The listing builds one solid part. Answer for the finished solid, in the listing's coordinates (mm). A direction names the side the tool comes from. Give positions to 0.01 mm unless a question says otherwise; leave off trailing zeros. Write each loop counter-clockwise with the first axis right and the second up, starting at its lowest first coordinate (ties: lowest second). Pieces come first, ordered by that corner, then holes. Notation, with made-up numbers: (-39, 63) - (-35, 63) arc R12 ccw to (-35, 81) - close; hole circle Ø9 at (79.5, 70). An arc over 180 degrees is marked (long way). Return JSON: item names as keys, results as strings.
from build123d import *

# Parameters (mm, degrees)
SKICA1_W                 = 54.3
SKICA1_H                 = 104.3
SKICA1_W_2               = 51
SKICA1_H_2               = 101
P_IDAT_VYSUNUT_M1_DEPTH  = 1.2
SKICA2_W                 = 54.3
SKICA2_H                 = 104.3
P_IDAT_VYSUNUT_M2_DEPTH  = 20
SKICA3_R                 = 1.5
ODEBRAT_VYSUNUT_M1_DEPTH = 118.085631057
SKICA5_W                 = 8
SKICA5_H                 = 4
ODEBRAT_VYSUNUT_M2_DEPTH = 2
SKICA6_W                 = 10
SKICA6_H                 = 4
ODEBRAT_VYSUNUT_M3_DEPTH = 5
SKICA9_W                 = 15
SKICA9_H                 = 5
P_IDAT_VYSUNUT_M4_DEPTH  = 2
ZKOSEN_1_SIZE            = 2
SKICA10_W                = 15
SKICA10_H                = 5
P_IDAT_VYSUNUT_M5_DEPTH  = 3
ZKOSEN_2_SIZE            = 3
ZAOBLIT2_R               = 1
ZAOBLIT3_R               = 2
ODEBRAT_VYSUNUT_M5_DEPTH = 12.5
SKICA12_R                = 1.5
ODEBRAT_VYSUNUT_M6_DEPTH = 118.296568577


with BuildPart() as part:
    # Skica1 → Přidat vysunutím1 (new body)
    with BuildSketch(Plane(origin=(0, 0, 0), x_dir=(1, 0, 0), z_dir=(0, 1, 0))):
        with Locations((25.5, 50.5)):
            Rectangle(SKICA1_W, SKICA1_H)
        with Locations((25.5, 50.5)):
            Rectangle(SKICA1_W_2, SKICA1_H_2, mode=Mode.SUBTRACT)
    extrude(amount=P_IDAT_VYSUNUT_M1_DEPTH)

    # Skica2 → Přidat vysunutím2 (add)
    # profile 1 of 5: a face of its own
    with BuildSketch(Plane.XZ):
        with Locations((25.5, -50.5)):
            Rectangle(SKICA2_W, SKICA2_H)
        Polygon((0, -8), (0, 0), (8, 0), (43, 0), (51, 0), (51, -8), (51, -93), (51, -101), (43, -101), (8, -101), (0, -101), (0, -93), align=None, mode=Mode.SUBTRACT)
    # profile 2 of 5: a face of its own
    with BuildSketch(Plane.XZ):
        with BuildLine():
            Line((8, 0), (0, 0))
            Line((0, 0), (0, -8))
            ThreePointArc((0, -8), (5.656854249, -5.656854249), (8, 0))
        make_face()
    # profile 3 of 5: a face of its own
    with BuildSketch(Plane.XZ):
        with BuildLine():
            ThreePointArc((8, -101), (5.656854249, -95.343145751), (0, -93))
            Line((0, -93), (0, -101))
            Line((0, -101), (8, -101))
        make_face()
    # profile 4 of 5: a face of its own
    with BuildSketch(Plane.XZ):
        with BuildLine():
            Line((51, -101), (51, -93))
            ThreePointArc((51, -93), (45.343145751, -95.343145751), (43, -101))
            Line((43, -101), (51, -101))
        make_face()
    # profile 5 of 5: a face of its own
    with BuildSketch(Plane.XZ):
        with BuildLine():
            Line((51, 0), (43, 0))
            ThreePointArc((43, 0), (45.343145751, -5.656854249), (51, -8))
            Line((51, -8), (51, 0))
        make_face()
    extrude(amount=P_IDAT_VYSUNUT_M2_DEPTH)

    # Skica3 → Odebrat vysunutím1 (cut, through all)
    with BuildSketch(Plane(origin=(0, 0, 0), x_dir=(1, 0, 0), z_dir=(0, 1, 0))):
        with Locations(Location((3.5, 97.5, 0), (0, 0, 270))):
            Circle(SKICA3_R)
        with Locations(Location((47.5, 97.5, 0), (0, 0, 270))):
            Circle(SKICA3_R)
        with Locations(Location((47.5, 3.5, 0), (0, 0, 270))):
            Circle(SKICA3_R)
    extrude(amount=-ODEBRAT_VYSUNUT_M1_DEPTH, mode=Mode.SUBTRACT)

    # Skica5 → Odebrat vysunutím2 (cut)
    with BuildSketch(Plane(origin=(0, 0, 0), x_dir=(0, 0, -1), z_dir=(1, 0, 0))):
        with Locations((27, -8.6)):
            Rectangle(SKICA5_W, SKICA5_H)
    extrude(amount=-ODEBRAT_VYSUNUT_M2_DEPTH, mode=Mode.SUBTRACT)

    # Skica6 → Odebrat vysunutím3 (cut, symmetric)
    with BuildSketch(Plane(origin=(0, 0, 0), x_dir=(-1, 0, 0), z_dir=(0, 0, -1))):
        with Locations((-12, -9.2)):
            Rectangle(SKICA6_W, SKICA6_H)
    extrude(amount=ODEBRAT_VYSUNUT_M3_DEPTH, both=True, mode=Mode.SUBTRACT)

    # Skica9 → Přidat vysunutím4 (add)
    with BuildSketch(Plane.ZY.offset(-51)):
        with Locations((-56.5, -2.5)):
            Rectangle(SKICA9_W, SKICA9_H)
    extrude(amount=P_IDAT_VYSUNUT_M4_DEPTH)

    # Zkosení1
    zkosen_1_edges = [part.edges().sort_by_distance(p)[0] for p in [
        (49, -5, -56.5),
    ]]
    chamfer(zkosen_1_edges, length=ZKOSEN_1_SIZE - 0.0001)  # a hair under: the kernel refuses the full size

    # Skica10 → Přidat vysunutím5 (add)
    with BuildSketch(Plane(origin=(0, 0, 0), x_dir=(0, 0, -1), z_dir=(1, 0, 0))):
        with Locations((70.5, -2.5)):
            Rectangle(SKICA10_W, SKICA10_H)
    extrude(amount=P_IDAT_VYSUNUT_M5_DEPTH)

    # Zkosení2
    zkosen_2_edges = [part.edges().sort_by_distance(p)[0] for p in [
        (3, -5, -70.5),
    ]]
    chamfer(zkosen_2_edges, length=ZKOSEN_2_SIZE - 0.0001)  # a hair under: the kernel refuses the full size

    # Zaoblit2
    zaoblit2_edges = [part.edges().sort_by_distance(p)[0] for p in [
        (7, -11.2, -1.111491673),
        (17, -11.2, 0.825),
    ]]
    fillet(zaoblit2_edges, radius=ZAOBLIT2_R)

    # Zaoblit3
    zaoblit3_edges = [part.edges().sort_by_distance(p)[0] for p in [
        (-1.65, -9.4, -102.65),
        (52.65, -9.4, -102.65),
        (52.65, -9.4, 1.65),
        (-1.65, -9.4, 1.65),
    ]]
    fillet(zaoblit3_edges, radius=ZAOBLIT3_R)

    # Skica11 → Odebrat vysunutím5 (cut)
    with BuildSketch(Plane(origin=(0, 0, 0), x_dir=(1, 0, 0), z_dir=(0, 1, 0))):
        with BuildLine():
            Line((0, 8), (0, 0))
            Line((0, 0), (8, 0))
            ThreePointArc((8, 0), (5.656854249, 5.656854249), (0, 8))
        make_face()
    extrude(amount=-ODEBRAT_VYSUNUT_M5_DEPTH, mode=Mode.SUBTRACT)

    # Skica12 → Odebrat vysunutím6 (cut, through all)
    with BuildSketch(Plane.XZ.offset(20)):
        with Locations(Location((3.5, -3.5, 0), (0, 0, 270))):
            Circle(SKICA12_R)
    extrude(amount=-ODEBRAT_VYSUNUT_M6_DEPTH, mode=Mode.SUBTRACT)


solid = part.part
Item 1: For faces 4 (the face through (49, 0, -99)), 5 (the face through (1, -2, -78)), 6 (the face through (-1, 1.2, -51)), determine the directions among +Z, -Z, +X, -X, +Y, -Y from which every point of the face is accessible in a straight line to the end or side of a thin tool.
Answer below:
{"face 4": "+Y", "face 5": "+Y, -Y", "face 6": "+Z, -Z, +X, -X, +Y"}
Item 2: A cutting plane is placed at C-C on x = 9.5. Determine the outline of the cut face in (y, z).
Answer below:
{"outline": "(-20, -102.65) - (1.2, -102.65) - (1.2, -101) - (-20, -101) - close; (-20, 0) - (-11.2, 0) - (-11.2, 1.65) - (-20, 1.65) - close; (-7.2, 0) - (1.2, 0) - (1.2, 1.65) - (-7.2, 1.65) - close"}
Item 3: Flat-ended cylindrical pins translate along their axes: P1, Ø1.8, axis at y = -9, z = 1, coming from the +X side; P2, Ø5, axis at x = 47.5, z = -97.5, coming from the -Y side; P3, Ø6.5, axis at x = 45, z = -4, coming from the +Y side; P4, Ø0.5, axis at x = -1, y = -8, coming from the -Z side. Find the tip coordinate at first contact, or state that the pin passes through.
Answer below:
{"P1": "stops at x = 52.6", "P2": "stops at y = -20", "P3": "stops at y = 0", "P4": "stops at z = -102.32"}
Item 4: The mould has two halves that part along X. Classify faces 1 (the face through (-1.08, -9.55, -102.05)), 2 (the face through (2.17, -9.86, -96.81)), 3 (the face through (52.05, -9.25, 1.08)): +X half, -X half, draft (parallel to the pull), parting line (faces both ways), or undercut.
Answer below:
{"face 1": "-X half", "face 2": "undercut", "face 3": "+X half"}
Item 5: Consider L1, parallel to X at y = -10, z = -68.5; L2, parallel to Z at x = 26, y = -12.75; L3, parallel to X at y = -15.25, z = -97.5. Determine where each line is inside the solid, lowest interval first.
Answer below:
{"L1": "x = -1.65 to 0, 51 to 52.65", "L2": "z = -102.65 to -101, 0 to 1.65", "L3": "x = -1.65 to 2, 5 to 7.19, 43.81 to 46, 49 to 52.65"}
Item 6: A cutting plane is placed at D-D on x = 20. Determine the outline of the cut face in (y, z), then the cut area to 3 significant figures.
Answer below:
{"outline": "(-20, -102.65) - (1.2, -102.65) - (1.2, -101) - (-20, -101) - close; (-20, 0) - (1.2, 0) - (1.2, 1.65) - (-20, 1.65) - close", "area": "70.0 mm²"}
Item 7: A cutting plane is placed at A-A on y = -9. Determine the outline of the cut face in (x, z), then the cut area to 3 significant figures.
Answer below:
{"outline": "(-1.65, -100.65) arc R2 ccw to (0.35, -102.65) - (50.65, -102.65) arc R2 ccw to (52.65, -100.65) - (52.65, -0.35) arc R2 ccw to (50.65, 1.65) - (17, 1.65) - (17, 0) - (43, 0) arc R8 ccw to (51, -8) - (51, -93) arc R8 ccw to (43, -101) - (8, -101) arc R8 ccw to (0, -93) - (0, -31) - (-1.65, -31) - close; (-1.65, -23) - (0, -23) - (0, 0) - (7, 0) - (7, 1.65) - (0.35, 1.65) arc R2 ccw to (-1.65, -0.35) - close; hole circle Ø3 at (3.5, -97.5); hole circle Ø3 at (47.5, -97.5); hole circle Ø3 at (47.5, -3.5)", "area": "609 mm²"}
